Design review of the part built by this model. Coordinates are the model's own, in mm. A direction names the side the tool comes from. Coordinates: 2 decimals unless noted, no trailing zeros. Write each loop counter-clockwise with the first axis right and the second up, starting at its lowest first coordinate (ties: lowest second). Pieces come first, ordered by that corner, then holes. Notation, with made-up numbers: (-20, 49.25) - (17, 49.25) arc R18 cw to (17, 66.25) - close; hole circle Ø6 at (22.25, -31). An arc over 180 degrees is marked (long way). One line per item, written item: value.
from build123d import *

# Parameters (mm, degrees)
SKETCH1_R           = 1
SKETCH1_R_2         = 3
SKETCH1_R_3         = 2.9
SKETCH1_W           = 2.7
SKETCH1_H           = 4.614285715
SKETCH1_H_2         = 4.614285714
BOSS_EXTRUDE1_DEPTH = 2.7


with BuildPart() as part:
    # Sketch1 → Boss-Extrude1 (new body)
    with BuildSketch(Plane(origin=(0, 0, 0), x_dir=(0, 0, -1), z_dir=(1, 0, 0))):
        Polygon((10.714285714, -32.5), (6.428571429, -32.5), (6.428571429, -29.8), (2.142857143, -29.8), (2.142857143, -32.5), (-2.142857143, -32.5), (-2.142857143, -29.8), (-6.428571429, -29.8), (-6.428571429, -32.5), (-10.714285714, -32.5), (-10.714285714, -29.8), (-15, -29.8), (-15, 2.5), (-32.5, 2.5), (-32.5, 32.5), (32.5, 32.5), (32.5, 2.5), (15, 2.5), (15, -29.8), (10.714285714, -29.8), align=None)
        with Locations((21.25, 26.25)):
            Circle(SKETCH1_R, mode=Mode.SUBTRACT)
        with Locations((21.25, 8.75)):
            Circle(SKETCH1_R, mode=Mode.SUBTRACT)
        with Locations((-21.25, 8.75)):
            Circle(SKETCH1_R, mode=Mode.SUBTRACT)
        with Locations((-21.25, 26.25)):
            Circle(SKETCH1_R, mode=Mode.SUBTRACT)
        with Locations((-27.5, 17.5)):
            Circle(SKETCH1_R_2, mode=Mode.SUBTRACT)
        with Locations((27.5, 17.5)):
            Circle(SKETCH1_R_3, mode=Mode.SUBTRACT)
        with Locations((0, -4.421428571)):
            Rectangle(SKETCH1_W, SKETCH1_H, mode=Mode.SUBTRACT)
        with Locations((0, -13.65)):
            Rectangle(SKETCH1_W, SKETCH1_H_2, mode=Mode.SUBTRACT)
        with Locations((0, -22.878571429)):
            Rectangle(SKETCH1_W, SKETCH1_H, mode=Mode.SUBTRACT)
        Polygon((0, 7.5), (14.5, 7.5), (22.5, 13.5), (22.5, 21.5), (14.5, 27.5), (-14.5, 27.5), (-22.5, 21.5), (-22.5, 13.5), (-14.5, 7.5), align=None, mode=Mode.SUBTRACT)
    extrude(amount=-BOSS_EXTRUDE1_DEPTH)


solid = part.part
1. Consider section C-C, the plane y = 17.5. Write out the cut boundary in (x, z), then the cut area to 3 significant figures.
Answer block:
outline: (-2.7, -32.5) - (0, -32.5) - (0, -30.4) - (-2.7, -30.4) - close; (-2.7, -24.6) - (0, -24.6) - (0, -22.5) - (-2.7, -22.5) - close; (-2.7, 22.5) - (0, 22.5) - (0, 24.5) - (-2.7, 24.5) - close; (-2.7, 30.5) - (0, 30.5) - (0, 32.5) - (-2.7, 32.5) - close
area: 22.1 mm^2
2. Consider section A-A, the plane z = 27.5. Write out the cut boundary in (x, y), then the cut area to 3 significant figures.
Answer block:
outline: (-2.7, 2.5) - (0, 2.5) - (0, 14.5) - (-2.7, 14.5) - close; (-2.7, 20.5) - (0, 20.5) - (0, 32.5) - (-2.7, 32.5) - close
area: 64.8 mm^2
3. Insertion check: pin 1 Ø0.8 at (x, y) = (-1, -31.5) entering from -Z; pin 2 Ø0.8 at (x, y) = (-1.5, -31) entering from +Z; pin 3 Ø1.4 at (x, z) = (-1, -5.5) entering from -Y. Each pin has a flat end and moves straight along its axis. Give the tip position at first contact, or say it passes through.
Answer block:
pin 1: stops at z = -10.71
pin 2: stops at z = 10.71
pin 3: stops at y = -29.8
4. Wall thickness on line 1 along Y through (x, z) = (-1.1, 27.5); line 2 along Y through (x, z) = (-2.25, 21.5); line 3 along Y through (x, z) = (-0.2, 11.5): over which ranges is each line inside the solid? List them lowest first.
Answer block:
line 1: y = 2.5 to 14.5, 20.5 to 32.5
line 2: y = 2.5 to 7.78, 9.72 to 12.75, 22.25 to 25.28, 27.22 to 32.5
line 3: y = -29.8 to 7.5, 27.5 to 32.5
5. For faces 1 (the face through (-1, -29.8, 13)), 2 (the face through (-1, -29.8, -13)), 3 (the face through (-1, -23, -1.35)), list the 3-axis set-ups (+Z, -Z, +X, -X, +Y, -Y) from which the entire face can be reached by the end or side of a thin tool; tool diameter is ignored.
Answer block:
face 1: +Z, +X, -X, -Y
face 2: -Z, +X, -X, -Y
face 3: +X, -X
6. Consider section B-B, the plane y = -3. Write out the cut boundary in (x, z), then the cut area to 3 significant figures.
Answer block:
outline: (-2.7, -15) - (0, -15) - (0, -1.35) - (-2.7, -1.35) - close; (-2.7, 1.35) - (0, 1.35) - (0, 15) - (-2.7, 15) - close
area: 73.7 mm^2
7. Mouldability with a two-part tool opening along Z and no side actions: class faces 4 (the face through (-1.33, 9.74, -21.12)), 5 (the face through (0, 0, 0)), 6 (the face through (-1, -13, -15)) as released by +Z, released by -Z, zero draft, split by the parting line, or undercut.
Answer block:
face 4: undercut
face 5: zero draft
face 6: released by -Z
8. Consider section D-D, the plane z = -21.25. Write out the cut boundary in (x, y), then the cut area to 3 significant figures.
Answer block:
outline: (-2.7, 2.5) - (0, 2.5) - (0, 7.75) - (-2.7, 7.75) - close; (-2.7, 9.75) - (0, 9.75) - (0, 12.56) - (-2.7, 12.56) - close; (-2.7, 22.44) - (0, 22.44) - (0, 25.25) - (-2.7, 25.25) - close; (-2.7, 27.25) - (0, 27.25) - (0, 32.5) - (-2.7, 32.5) - close
area: 43.5 mm^2
